Autodesk Inventor part; units mm, degrees
ref_plane "YZ Plane" through (0, 0, 0) normal (1, 0, 0) x (0, 1, 0)
ref_plane "XZ Plane" through (0, 0, 0) normal (0, 1, 0) x (-1, 0, 0)
ref_plane "XY Plane" through (0, 0, 0) normal (0, 0, 1) x (1, 0, 0)
sketch "Sketch1" plane through (0, 0, 0) normal (0, 0, 1) x (1, 0, 0)
  line L0 (0, 4.675) -> (0, -4.675)
  line L1 (0, -4.675) -> (0.75, -4.675)
  line L2 (0.75, -4.675) -> (1, -4.425)
  line L3 (1, -4.425) -> (1, 3.225)
  line L4 (1.1, 3.325) -> (1.9, 3.325)
  line L5 (1.9, 3.325) -> (1.9, 4.525)
  line L6 (1.75, 4.675) -> (0, 4.675)
  arc A0 (1.1, 3.325) -> (1, 3.225) centre (1.1, 3.225) ccw
  line L7 (1.75, 4.675) -> (1.9, 4.525)
  point P0 (0, 0)
  point P1 (1.9, 4.675)
  point P2 (0, 0)
  dimension "d0" = 3.8
  dimension "d1" = 1.35
  dimension "d3" = 2
  dimension "d4" = 2.2
  dimension "d5" = 135
  dimension "d6" = 0.25
  dimension "d7" = 8
  dimension "d18" = 0.15
  dimension "d22" = 0.15
revolve "Revolution1" add sketch "Sketch1" angle 360 about axis through (0, 4.675, 0) along (0, -1, 0)
sketch "Sketch2" plane through (0, 4.675, 0) normal (0, 1, 0) x (1, 0, 0)
  line L0 (0, -0.7506) -> (-0.65, -0.3753)
  line L1 (-0.65, -0.3753) -> (-0.65, 0.3753)
  line L2 (-0.65, 0.3753) -> (0, 0.7506)
  line L3 (0, 0.7506) -> (0.65, 0.3753)
  line L4 (0.65, 0.3753) -> (0.65, -0.3753)
  line L5 (0.65, -0.3753) -> (0, -0.7506)
  point P0 (0, 0)
  point P1 (0, 0)
  dimension "d11" = 1.3
extrude "Extrusion1" cut sketch "Sketch2" against normal blind 1
thread "Thread1"
sketch "Sketch3" plane through (0, 0, 0) normal (1, 0, 0) x (0, 1, 0)
  line L0 (4.675, 0.7506) -> (4.675, 0.3753)
  line L1 (4.675, 0.7506) -> (4.175, 0.2506)
  line L2 (4.175, 0.2506) -> (4.675, 0.2506)
  line L3 (4.675, 0.2506) -> (4.675, 0.7506)
  line L4 (-0.7, 0) -> (4.2, 0)
  point P0 (0, 0)
  dimension "d16" = 0.5
revolve "Revolution2" cut sketch "Sketch3" angle 360 about axis through (0, -10, 0) along (0, 1, 0)
equation "\"d22\" = d18"
properties part number "48-0280" material "Stainless Steel"
Could you check a few things on this model? Use its own coordinates, in mm. A direction names the side the tool comes from. Coordinates: 2 decimals unless noted, no trailing zeros. Write each loop counter-clockwise with the first axis right and the second up, starting at its lowest first coordinate (ties: lowest second). Pieces come first, ordered by that corner, then holes. Notation, with made-up numbers: (76, 52.5) -> (116, 52.5) arc R19 ccw to (116, 59.5) -> close; hole circle Ø5 at (82, 15.5). An arc over 180 degrees is marked (long way). Write item = value, one per line. Start each with the question number.
(1) I need wall thicknesses on line 1 (Y direction, x = -0.8, z = 1.15) (3 decimals); line 2 (Y direction, x = -0.1, z = -0.3) (3 decimals); line 3 (Z direction, x = -0.1, y = -1.75). Which ranges of each line are inside material? Lowest first, please. Write a range as [from, to].
(2) Will these pins go through, and if not, where does the flat tip stop? pin 1 (2 mm diameter, centred on x = 0.5, y = 0, fed in from -Z); pin 2 (1.5 mm diameter, centred on y = -0.5, z = 0.5, fed in from +X); pin 3 (1.4 mm diameter, centred on x = 0, z = 0, fed in from +Y).
(3) We'd pull the mould along Z, two halves only. Please class faces 1 (the face through (-1.9, 3.93, -0.08)), 2 (the face through (0, 3.675, 0)), 3 (the face through (0, 4.675, -1)): released by +Z, released by -Z, zero draft, split by the parting line, or undercut.
(4) I want a section at B-B (y = 0). Please give me the cut outline in (x, z), plus the area to 3 significant figures.
(5) I want a section at A-A (z = 0). Please give me the cut outline in (x, y) (3 decimals), plus the area to 3 significant figures.
(6) Which directions (+Z, -Z, +X, -X, +Y, -Y) give clear straight access to the entire face, cutting with the end or side of a thin tool? Please do faces 4 (the face through (0, -4.675, 0)), 5 (the face through (1, 3.325, -1)).
Result set:
q1.line_1 = [3.325, 4.675]
q1.line_2 = [-4.675, 3.675]
q1.line_3 = [-0.99, 0.99]
q2.pin_1 = -1
q2.pin_2 = 1
q2.pin_3 = 4.62
q3.face_1 = split by the parting line
q3.face_2 = undercut
q3.face_3 = zero draft
q4.outline = circle Ø2 at (0, 0)
q4.area = 3.14 mm2
q5.outline = (-1.9, 3.325) -> (-1.1, 3.325) arc R0.1 cw to (-1, 3.225) -> (-1, -4.425) -> (-0.75, -4.675) -> (0.75, -4.675) -> (1, -4.425) -> (1, 3.225) arc R0.1 cw to (1.1, 3.325) -> (1.9, 3.325) -> (1.9, 4.525) -> (1.75, 4.675) -> (0.751, 4.675) -> (0.65, 4.574) -> (0.65, 3.675) -> (-0.65, 3.675) -> (-0.65, 4.574) -> (-0.751, 4.675) -> (-1.75, 4.675) -> (-1.9, 4.525) -> close
q5.area = 19.7 mm2
q6.face_4 = +Z, -Z, +X, -X, -Y
q6.face_5 = -Y
